For this review, take the finished solid that the model builds, in its own axes (mm). Face numbers are marked on the shaded views. Give positions to 0.01 mm unless a question says otherwise; leave off trailing zeros. Write each loop counter-clockwise with the first axis right and the second up, starting at its lowest first coordinate (ties: lowest second). Pieces come first, ordered by that corner, then holes. Notation, with made-up numbers: M -33.5,58 L 6.5,58 A29 cw 6.5,82 Z; hole C 78,10 d1. An arc over 180 degrees is marked long. Use one line per item in the form item = value. Start each with the question number.
Q1. For probe 1 along Y at (x, z) = (0, 3.5); probe 2 along Y at (x, z) = (0, -2); probe 3 along Z at (x, y) = (5.5, -6), list the stretches that pass through material, from the lowest coordinate up. Write a range as [from, to].
Q2. Consider section D-D on z = 3. Write out the cut boundary in (x, y), and give its area (3 significant figures).
Q3. Consider section C-C on z = -2.5. Write out the cut boundary in (x, y).
Q4. Consider section A-A on y = 0. Write out the cut boundary in (x, z).
Q5. Clearance check with flat-ended pins moving along their axes: pin 1 Ø5 at (x, y) = (2, -2.5) entering from +Z; pin 2 Ø1.5 at (x, z) = (1, 1.5) entering from -Y. State where each tip first meets the part, or that it passes through.
Q6. Mouldability with a two-part tool opening along X and no side actions: class the marked faces 1, 2 and 3 as released by +X, released by -X, zero draft, split by the parting line, or undercut.
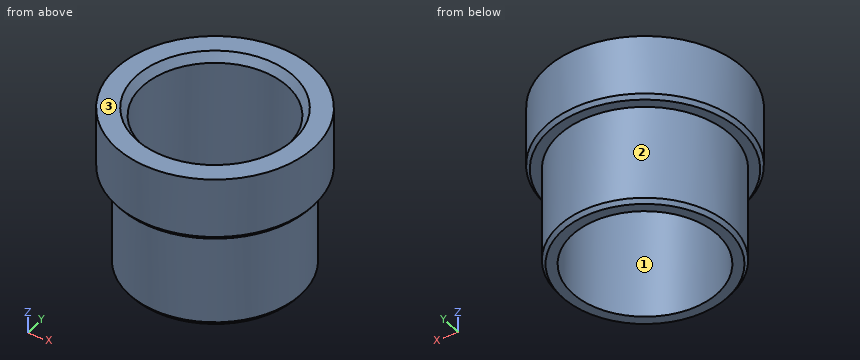
```python
from build123d import *
from OCP.BRepFilletAPI import BRepFilletAPI_MakeChamfer

# Parameters (mm, degrees)
CHAMFER1_SIZE  = 0.7112
CHAMFER1_SIZE2 = 0.53592764
CHAMFER2_SIZE  = 0.3556
CHAMFER2_SIZE2 = 0.26796382


with BuildPart() as part:
    # Sketch2 → Revolve1 (revolve)
    with BuildSketch(Plane(origin=(0, 0, 0), x_dir=(0, 0, -1), z_dir=(1, 0, 0)), mode=Mode.PRIVATE) as revolve1_sk:
        Polygon((7.112, 6.35), (7.112, 7.493), (-1.524, 7.493), (-1.524, 8.636), (-7.112, 8.636), (-7.112, 6.35), align=None)
    revolve(revolve1_sk.sketch.rotate(Axis((0, 0, -7.112), (0, 0, 1)), 90), axis=Axis((0, 0, -7.112), (0, 0, 1)))

    # Chamfer1
    chamfer1_edges = [part.edges().sort_by_distance(p)[0] for p in [
        (6.35, 0, 7.112),
    ]]
    chamfer1_side = [part.faces().sort_by_distance(p)[0] for p in [
        (6.35, 0, 0),
    ]]
    chamfer(chamfer1_edges, length=CHAMFER1_SIZE, length2=CHAMFER1_SIZE2, reference=chamfer1_side[0])

    # Chamfer2: one chamfer whose edges measure the first distance from different faces: ONE call of the kernel's chamfer builder (chamfer() names one face for all edges)
    chamfer2_edges_1 = [part.edges().sort_by_distance(p)[0] for p in [
        (8.636, 0, 1.524),
    ]]
    chamfer2_side_1 = [part.faces().sort_by_distance(p)[0] for p in [
        (8.636, 0, 4.318),
    ]]
    chamfer2_edges_2 = [part.edges().sort_by_distance(p)[0] for p in [
        (7.493, 0, -7.112),
    ]]
    chamfer2_side_2 = [part.faces().sort_by_distance(p)[0] for p in [
        (7.493, 0, -2.794),
    ]]
    chamfer2 = BRepFilletAPI_MakeChamfer(part.part.solid().wrapped)
    for e in chamfer2_edges_1:
        chamfer2.Add(CHAMFER2_SIZE, CHAMFER2_SIZE2, e.wrapped, chamfer2_side_1[0].wrapped)  # the first distance lies on this face
    for e in chamfer2_edges_2:
        chamfer2.Add(CHAMFER2_SIZE, CHAMFER2_SIZE2, e.wrapped, chamfer2_side_2[0].wrapped)  # the first distance lies on this face
    add(Compound.cast(chamfer2.Shape()), mode=Mode.REPLACE)


solid = part.part
```
Working result:
q1.probe_1 = [-8.64, -6.35], [6.35, 8.64]
q1.probe_2 = [-7.49, -6.35], [6.35, 7.49]
q1.probe_3 = [1.52, 7.11]
q2.outline = C 0,0 d17.27; hole C 0,0 d12.7
q2.area = 108 mm²
q3.outline = C 0,0 d14.99; hole C 0,0 d12.7
q4.outline = M -8.64,1.88 L -8.37,1.52 L -7.49,1.52 L -7.49,-6.76 L -7.23,-7.11 L -6.35,-7.11 L -6.35,6.4 L -6.89,7.11 L -8.64,7.11 Z; M 6.35,-7.11 L 7.23,-7.11 L 7.49,-6.76 L 7.49,1.52 L 8.37,1.52 L 8.64,1.88 L 8.64,7.11 L 6.89,7.11 L 6.35,6.4 Z
q5.pin_1 = through
q5.pin_2 = -8.63
q6.face_1 = undercut
q6.face_2 = split by the parting line
q6.face_3 = zero draft
